CAD build for the part. Positions are in the model's coordinates, mm. A direction names the side the tool comes from. Round coordinates to 2 decimals unless told otherwise and drop trailing zeros. Loops run counter-clockwise (first coordinate to the right, second up) from the corner with the lowest first, then second, coordinate; pieces in that order, holes last. Notation, with made-up numbers: M -17.75,71.5 L 29.25,71.5 A16 cw 29.25,100.5 Z; hole C -9.75,66 d5. An arc over 180 degrees is marked long. Use one line per item in the form item = value.
from build123d import *

# Parameters (mm, degrees)
SKETCH_W        = 23
SKETCH_H        = 23.82
PAD_DEPTH       = 6
FILLET_R        = 3
POCKET_DEPTH    = 1
SKETCH001_W     = 40
SKETCH001_H     = 40
SKETCH001_R     = 11.45
POCKET001_DEPTH = 5
SKETCH004_R     = 7.95
POCKET002_DEPTH = 5
SKETCH006_R     = 1.75
HOLE_DEPTH      = 6.001
SKETCH007_R     = 2.75
POCKET004_DEPTH = 5
SKETCH008_R     = 1.5
HOLE001_DEPTH   = 25


with BuildPart() as part:
    # Sketch → Pad (new body)
    with BuildSketch(Plane.XY):
        Rectangle(SKETCH_W, SKETCH_H)
    extrude(amount=PAD_DEPTH)

    # Fillet
    fillet_edges = [part.edges().sort_by_distance(p)[0] for p in [
        (11.5, -11.91, 3),
        (-11.5, -11.91, 3),
        (11.5, 11.91, 3),
        (-11.5, 11.91, 3),
    ]]
    fillet(fillet_edges, radius=FILLET_R)

    # Sketch003 → Pocket (cut)
    with BuildSketch(Plane(origin=(0, 0, 0), x_dir=(1, 0, 0), z_dir=(0, 0, -1))):
        with BuildLine():
            ThreePointArc((4, -8.5), (5.75, -6.75), (4, -5))
            Line((4, -5), (-3.12, -5))
            ThreePointArc((-3.12, -5), (-4.87, -6.75), (-3.12, -8.5))
            Line((4, -8.5), (-3.12, -8.5))
        make_face()
        with BuildLine():
            ThreePointArc((2.38, 5.01), (4.13, 6.76), (2.38, 8.51))
            Line((2.38, 8.51), (-2.34, 8.51))
            ThreePointArc((-2.34, 8.51), (-4.09, 6.76), (-2.34, 5.01))
            Line((2.38, 5.01), (-2.34, 5.01))
        make_face()
    extrude(amount=-POCKET_DEPTH, mode=Mode.SUBTRACT)

    # Sketch001 (on Face6 of Pad) → Pocket001 (cut)
    with BuildSketch(Plane.XY.offset(6)):
        Rectangle(SKETCH001_W, SKETCH001_H)
        Circle(SKETCH001_R, mode=Mode.SUBTRACT)
    extrude(amount=-POCKET001_DEPTH, mode=Mode.SUBTRACT)

    # Sketch004 (on Face21 of Pocket001) → Pocket002 (cut)
    with BuildSketch(Plane(origin=(0, 0, 1), x_dir=(1, 0, 0), z_dir=(0, 0, -1))):
        with Locations((-0.007428, -0.004957)):
            Circle(SKETCH004_R)
    extrude(amount=-POCKET002_DEPTH, mode=Mode.SUBTRACT)

    # Sketch006 → Hole (cut, through all)
    with BuildSketch(Plane.XY.offset(6)):
        with Locations((-8.25, 8.25)):
            Circle(SKETCH006_R)
        with Locations((8.25, 8.25)):
            Circle(SKETCH006_R)
        with Locations((8.25, -8.25)):
            Circle(SKETCH006_R)
        with Locations((-8.25, -8.25)):
            Circle(SKETCH006_R)
    extrude(amount=-HOLE_DEPTH, mode=Mode.SUBTRACT)

    # Sketch007 → Pocket004 (cut)
    with BuildSketch(Plane.XY.offset(6)):
        with Locations((-8.293696, 8.188751)):
            Circle(SKETCH007_R)
        with Locations((8.293696, 8.188751)):
            Circle(SKETCH007_R)
        with Locations((8.293696, -8.188751)):
            Circle(SKETCH007_R)
        with Locations((-8.293696, -8.188751)):
            Circle(SKETCH007_R)
    extrude(amount=-POCKET004_DEPTH, mode=Mode.SUBTRACT)

    # Sketch008 (on Face6 of Pad) → Hole001 (cut)
    with BuildSketch(Plane.XY.offset(6)):
        Circle(SKETCH008_R)
    extrude(amount=-HOLE001_DEPTH, mode=Mode.SUBTRACT)


solid = part.part
1. Probe line 1 along Y through (x, z) = (0, 0.7); line 2 along Y through (x, z) = (-8.25, 0.2); line 3 along X through (y, z) = (7, 0.6). List the from-to ranges inside material, lowest first. Write a range as from..to.
Completed:
line_1 = -11.91..-8.51, -5.01..-1.5, 1.5..5, 8.5..11.91
line_2 = -11.91..-10, -6.5..6.5, 10..11.91
line_3 = -11.5..-9.47, -7.03..-4.85, 5.73..7.03, 9.47..11.5
2. Pull direction X, two halves, no side cores. Call faces 1 (the face through (10.64, 11.01, 0.51)), 2 (the face through (-1.5, 0.07, 0.51)), 3 (the face through (-11.5, -0.1, 0.5)), 4 (the face through (9.867, -8.92, 0.507)): +X half, -X half, draft (parallel to the pull), parting line (faces both ways), or undercut.
Completed:
face_1 = +X half
face_2 = undercut
face_3 = -X half
face_4 = undercut
3. Cut at C-C on y = -1. Write the cut outline in (x, z).
Completed:
outline = M -11.5,0 L -1.12,0 L -1.12,1 L -7.89,1 L -7.89,6 L -11.41,6 L -11.41,1 L -11.5,1 Z; M 1.12,0 L 11.5,0 L 11.5,1 L 11.41,1 L 11.41,6 L 7.88,6 L 7.88,1 L 1.12,1 Z
4. Cut at D-D on y = 2. Write the cut outline in (x, z).
Completed:
outline = M -11.5,0 L 11.5,0 L 11.5,1 L 11.27,1 L 11.27,6 L 7.69,6 L 7.69,1 L -7.7,1 L -7.7,6 L -11.27,6 L -11.27,1 L -11.5,1 Z
5. Tool access for faces 5 (the face through (-11.45, 0.09, 3.54)), 6 (the face through (-6.3, -6.295, 3.535)), 7 (the face through (0.5, 8.5, 0.5)): list every direction of +Z, -Z, +X, -X, +Y, -Y with a clear straight run to the whole face (end or side of a thin tool).
Completed:
face_5 = +Z, -X
face_6 = +Z
face_7 = -Z
6. Cut at A-A on x = 4.75. Write the cut outline in (y, z), and give its area (3 significant figures).
Completed:
outline = M -11.91,0 L 5.17,0 L 5.17,1 L -6.36,1 L -6.36,6 L -10.42,6 L -10.42,1 L -11.91,1 Z; M 6.37,1 L 8.33,1 L 8.33,0 L 11.91,0 L 11.91,1 L 10.42,1 L 10.42,6 L 6.37,6 Z
area = 61.1 mm2
7. Drop flat-ended pins along their axis: P1, Ø4.5, axis at x = -8.25, y = 8.25, coming from the +Z side; P2, Ø1.9, axis at x = -1.5, y = -7.5, coming from the -Z side; P3, Ø3, axis at x = -5, z = 5, coming from the -Y side. Give the stop position or say it passes through.
Completed:
P1 = 1
P2 = 1
P3 = -10.9
8. Cut at B-B on z = 4.05. Write the cut outline in (x, y), and give its area (3 significant figures).
Completed:
outline = M -9.81,-5.9 A2.75 cw -6.02,-9.74 A11.45 ccw 6.02,-9.74 A2.75 cw 9.81,-5.9 A11.45 ccw 9.81,5.9 A2.75 cw 6.02,9.74 A11.45 ccw -6.02,9.74 A2.75 cw -9.81,5.9 A11.45 ccw Z; hole C -0.01,0 d15.9
area = 173 mm2
